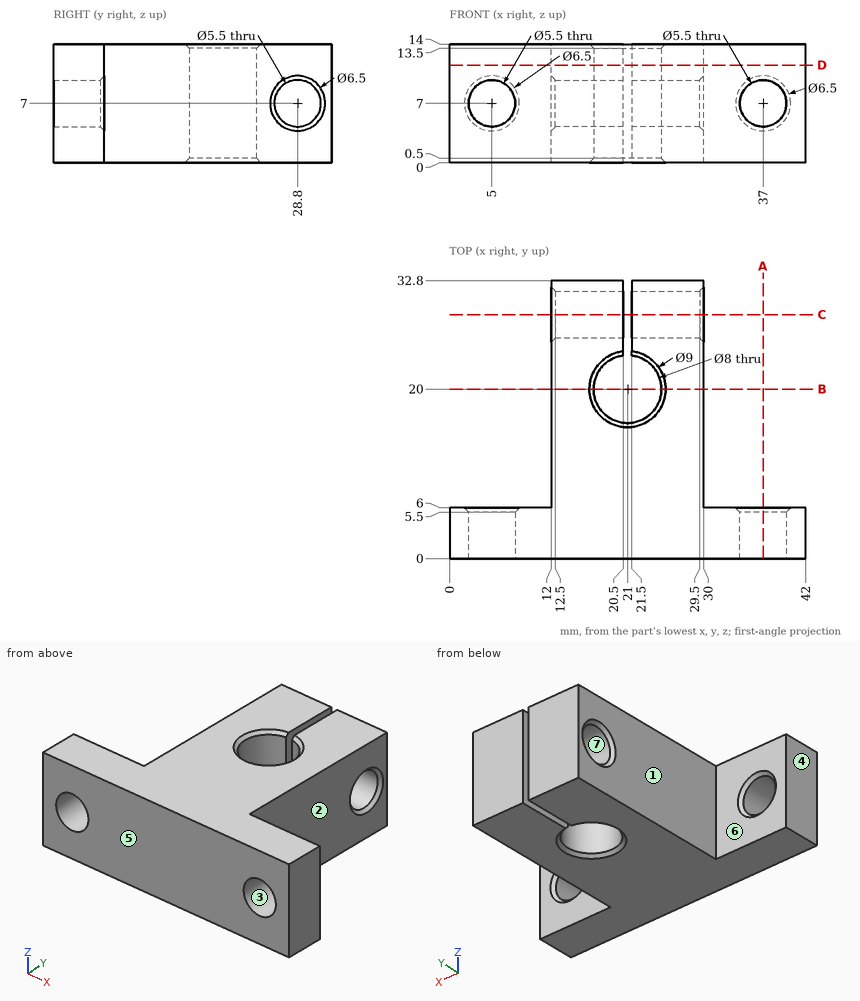
Study the drawing (mm; zero at the part's minimum x, y, z) and answer. A direction names the side the tool comes from. Coordinates: 2 decimals unless noted, no trailing zeros. Order: outer loops, then holes, each group sorted by start corner. A loop starts at its lowest first (then second) coordinate and runs counter-clockwise, first axis right, second up. Notation, with made-up numbers: (0.25, -4) -> (34.25, -4) arc R22 ccw to (34.25, 33) -> close; hole circle Ø11 at (81, 14.25). An arc over 180 degrees is marked (long way). Answer in a Markdown table with one row per item. Add a question column.
Item 1: Each of these flat-tipped pins is pushed along its axis until it touches: P1, Ø3.5, axis at y = 28.8, z = 7, coming from the -X side; P2, Ø7, axis at y = 29.5, z = 9.5, coming from the -X side; P3, Ø2.5, axis at y = 28, z = 5, coming from the +X side. Where does it stop, or does it pass through?
Item 2: Determine the mould class of the marked faces 4, 5, 6 and 7 for opening direction Y: +Y half, -Y half, draft (parallel to the pull), parting line (faces both ways), or undercut.
Item 3: Find section C-C (y = 28.8). Write down the section's boundary in (x, z), then the cut area to 3 significant figures.
Item 4: Find section A-A (x = 37). Write down the section's boundary in (y, z).
Item 5: Find the intervals of material crossed by L1, parallel to X at y = 25, z = 13.5; L2, parallel to Z at x = 5, y = 2.6; L3, parallel to X at y = 10, z = 4.5, in increasing order. Write a range as from..to.
Item 6: Find section D-D (z = 11.5). Write down the section's boundary in (x, y).
Item 7: Which of the six approach directions +Z, -Z, +X, -X, +Y, -Y give full straight-line access (tool end or side, diameter ignored) to the marked faces 1, 2 and 3?
Item 8: Find section B-B (y = 20). Write down the section's boundary in (x, z), then the cut area to 4 significant figures.
Result set:
| question | item | result |
|---|---|---|
| 1 | P1 | passes through |
| 1 | P2 | stops at x = 12 |
| 1 | P3 | stops at x = 30 |
| 2 | face 4 | draft |
| 2 | face 5 | -Y half |
| 2 | face 6 | +Y half |
| 2 | face 7 | undercut |
| 3 | outline | (12, 0) -> (20.5, 0) -> (20.5, 4.25) -> (12.5, 4.25) -> (12, 3.75) -> close; (12, 10.25) -> (12.5, 9.75) -> (20.5, 9.75) -> (20.5, 14) -> (12, 14) -> close; (21.5, 0) -> (30, 0) -> (30, 3.75) -> (29.5, 4.25) -> (21.5, 4.25) -> close; (21.5, 9.75) -> (29.5, 9.75) -> (30, 10.25) -> (30, 14) -> (21.5, 14) -> close |
| 3 | area | 144 mm² |
| 4 | outline | (0, 0) -> (6, 0) -> (6, 3.75) -> (5.5, 4.25) -> (0, 4.25) -> close; (0, 9.75) -> (5.5, 9.75) -> (6, 10.25) -> (6, 14) -> (0, 14) -> close |
| 5 | L1 | x = 12..20.5, 21.5..30 |
| 5 | L2 | z = 0..4.25, 9.75..14 |
| 5 | L3 | x = 12..30 |
| 6 | outline | (0, 0) -> (42, 0) -> (42, 6) -> (30, 6) -> (30, 32.8) -> (21.5, 32.8) -> (21.5, 23.97) arc R4 cw (long way) to (20.5, 23.97) -> (20.5, 32.8) -> (12, 32.8) -> (12, 6) -> (0, 6) -> close |
| 7 | face 1 | +Z, -Z, -X, +Y |
| 7 | face 2 | +Z, -Z, +X, +Y |
| 7 | face 3 | +Y, -Y |
| 8 | outline | (12, 0) -> (16.5, 0) -> (17, 0.5) -> (17, 13.5) -> (16.5, 14) -> (12, 14) -> close; (25, 0.5) -> (25.5, 0) -> (30, 0) -> (30, 14) -> (25.5, 14) -> (25, 13.5) -> close |
| 8 | area | 139.5 mm² |
